Autodesk Inventor part; units mm, degrees
ref_plane "XY Plane" through (0, 0, 0) normal (0, 0, 1) x (1, 0, 0)
sketch "Skizze1" plane through (0, 0, 0) normal (0, 0, 1) x (1, 0, 0)
  line L0 (-235, 150) -> (235, 150)
  line L1 (235, 150) -> (235, -150)
  line L2 (235, -150) -> (-235, -150)
  line L3 (-235, -150) -> (-235, 150)
  line L4 (-235, 150) -> (235, -150) construction
  line L5 (235, 150) -> (-235, -150) construction
  point P0 (0, 0)
  dimension "d0" = 300
  dimension "d1" = 470
extrude "Extrusion1" add sketch "Skizze1" against normal blind 15
sketch "Skizze2" plane through (0, 0, -15) normal (0, 0, -1) x (-1, 0, 0)
  line L0 (-235, -150) -> (235, -150)
  line L1 (235, -150) -> (235, 150)
  line L2 (235, 150) -> (-235, 150)
  line L3 (-235, 150) -> (-235, -150)
  point P0 (0, 0)
  point P1 (0, 40.5)
  point P2 (0, -40.5)
  dimension "d4" = 40.5
  dimension "d5" = 40.5
hole "Bohrung1" at (0, 40.5, -15) at (0, -40.5, -15) direction (0, 0, 1) diameter 9 end through all counterbore diameter 15 counterbore depth 9
pattern_linear "Rechteckige Anordnung1" count 2 spacing 200 along (1, 0, 0) count 2 spacing 200 along (-1, 0, 0) of "Bohrung1"
chamfer "Fasen1" distance 2 angle 45 4 edges at (235, -150, -7.5) (235, 150, -7.5) (-235, 150, -7.5) (-235, -150, -7.5)
chamfer "Fasen2" distance 2 angle 45 8 edges at (0, -150, -15) (0, -150, 0) (-235, 0, 0) (-235, 0, -15) (0, 150, 0) (0, 150, -15) (235, 0, 0) (235, 0, -15)
chamfer "Fasen3" distance 0.5 angle 45 6 edges at (-200, -48, -15) (-200, 33, -15) (0, -48, -15) (0, 33, -15) (200, -48, -15) (200, 33, -15)
chamfer "Fasen4" distance 0.5 angle 45 6 edges at (-200, -45, 0) (-200, 36, 0) (0, -45, 0) (0, 36, 0) (200, -45, 0) (200, 36, 0)
properties part number "Bodenplatte-Segment"
Build history of the part. All positions in model axes, mm. A direction names the side the tool comes from. Round coordinates to 2 decimals unless told otherwise and drop trailing zeros. Put each result on its own line as item: value.
Item 1: Two-plate mould, pull along Y, no slides. Class faces 1 (the face through (3, -150, -7)), 2 (the face through (-195.61, -41.48, -3.21)), 3 (the face through (-235, -2, -7)): pulls with the +Y half, pulls with the -Y half, needs draft (parallel to the pull), parting line crosses it, or undercut.
Here are the results:
face 1: pulls with the -Y half
face 2: undercut
face 3: needs draft
Item 2: Flat gauge pins, fed straight in: P1, Ø7.5, axis at x = -2, y = -37, coming from the -Z side; P2, Ø13.5, axis at x = 0, y = -40.5, coming from the -Z side. Where does each tip first touch, or does it go through?
Here are the results:
P1: stops at z = -14.78
P2: stops at z = -6
Item 3: Slice it at A-A, the plane x = 200. Count the separate pieces of the cut face and the enclosed holes in it, plus the area to 3 significant figures.
Here are the results:
separate pieces: 3
enclosed holes: 0
area: 4,110 mm^2
Item 4: Wall check: probe 1 along X at (y, z) = (-40.5, -4.5); probe 2 along X at (y, z) = (-40.5, -11.25); probe 3 along Y at (x, z) = (0, -3.35). Give the ranges that are in metal, low to high. Write a range as from..to.
Here are the results:
probe 1: x = -235..-204.5, -195.5..-4.5, 4.5..195.5, 204.5..235
probe 2: x = -235..-207.5, -192.5..-7.5, 7.5..192.5, 207.5..235
probe 3: y = -150..-45, -36..36, 45..150
Item 5: Tool access for faces 4 (the face through (0, 33, -10)), 5 (the face through (-1.352, 44.792, -3.212)): list every direction of +Z, -Z, +X, -X, +Y, -Y with a clear straight run to the whole face (end or side of a thin tool).
Here are the results:
face 4: -Z
face 5: +Z, -Z
